Could you check a few things on this model? Use its own coordinates, in mm. Round coordinates to 2 decimals unless told otherwise and drop trailing zeros. Order: outer loops, then holes, each group sorted by start corner. A loop starts at its lowest first (then second) coordinate and runs counter-clockwise, first axis right, second up.
```python
from build123d import *

# Parameters (mm, degrees)
F0_W     = 127.7268081903
F0_H     = 72.7801807225
F0_R     = 18.9582782215
F2_DEPTH = 39.37


# Not quite as in the source:
# - the program builds the solid bodies; features that only make, move or delete a surface that nothing else refers to are left out


with BuildPart() as f2:
    # F0 (on Front) → F2 (new body)
    with BuildSketch(Plane.XZ):
        with Locations((4.9403756857, 0.8434783667)):
            Rectangle(F0_W, F0_H)
        Circle(F0_R, mode=Mode.SUBTRACT)
    extrude(amount=F2_DEPTH)


solid = f2.part
```
Q1. For P1, Ø2, axis at x = 4.5, z = 16.5, coming from the +Y side, with a flat end and sliding along its axis, tell me the tip position at first contact or that it passes through.
Q2. Imagine slicing it at B-B, the plane z = 0. Please give me the cut outline in (x, y).
Q3. Imagine slicing it at C-C, the plane y = -18. Please give me the cut outline in (x, z).
Q4. I need wall thicknesses on L1, parallel to Z at x = 0, y = -14; L2, parallel to X at y = -16, z = -4.5; L3, parallel to X at y = -31.5, z = 14. Which ranges of each line are inside material? Lowest first, please.
Q5. We'd pull the mould along Z, two halves only. Please class faces 1 (the cylindrical face through (-4.11, -19.409, -18.507)), 2 (the flat face through (4, -19, -35.547)), 3 (the flat face through (68.804, -19, 0)), 4 (the flat face through (4, -19, 37.234)): released by +Z, released by -Z, zero draft, split by the parting line, or undercut.
Q6. Imagine slicing it at A-A, the plane x = 0. Please give me the cut outline in (y, z).
Filled in:
1. P1: passes through
2. outline: (-58.92, -39.37) - (-18.96, -39.37) - (-18.96, 0) - (-58.92, 0) - close; (18.96, -39.37) - (68.8, -39.37) - (68.8, 0) - (18.96, 0) - close
3. outline: (-58.92, -35.55) - (68.8, -35.55) - (68.8, 37.23) - (-58.92, 37.23) - close; hole circle Ø37.92 at (0, 0)
4. L1: z = -35.55 to -18.96, 18.96 to 37.23
4. L2: x = -58.92 to -18.42, 18.42 to 68.8
4. L3: x = -58.92 to -12.78, 12.78 to 68.8
5. face 1: undercut
5. face 2: released by -Z
5. face 3: zero draft
5. face 4: released by +Z
6. outline: (-39.37, -35.55) - (0, -35.55) - (0, -18.96) - (-39.37, -18.96) - close; (-39.37, 18.96) - (0, 18.96) - (0, 37.23) - (-39.37, 37.23) - close
